Geometry: final body of the model. Coordinates: model frame, mm. Face numbers are marked on the shaded views. A direction names the side the tool comes from. Give positions to 0.01 mm unless a question says otherwise; leave off trailing zeros. Write each loop counter-clockwise with the first axis right and the second up, starting at its lowest first coordinate (ties: lowest second). Pieces come first, ordered by that corner, then holes.
Q1. Cut plane D-D on z = 7.75. Return the cut outline in (x, y).
Q2. Cut plane C-C on x = 3.75. Return the cut outline in (y, z), plus the area to 3 significant figures.
Q3. Pin query (flat end, axial travel): pin 1 (2 mm diameter, centred on x = 4.5, y = 0, fed in from +Z); pin 2 (2 mm diameter, centred on x = 6.5, y = 3.5, fed in from +Z). Return the tip coordinate at first contact, or that it passes through.
Q4. Draft query along Z for the marked faces 3, 4 and 5. Return one class per face: pulls with the +Z half, pulls with the -Z half, needs draft (parallel to the pull), parting line crosses it, or undercut.
Q5. Line query: L1, parallel to X at y = -0.75, z = 10; L2, parallel to Z at x = 5.75, y = 4; L3, parallel to Z at x = 1, y = 3.75. Output: solid intervals per line, ascending.
Q6. Reachability of the marked faces 1 and 2 from +Z, -Z, +X, -X, +Y, -Y: full face, straight path, thin tool, end or side. Return the list, or none.
Q7. Cut plane B-B on z = 13.75. Return the cut outline in (x, y), plus the area to 3 significant figures.
Q8. Cut plane A-A on y = 0.25. Return the cut outline in (x, z).
```python
from build123d import *

# Parameters (mm, degrees)
SKETCH1_R           = 6
BOSS_EXTRUDE1_DEPTH = 2
SKETCH2_R           = 4.5
BOSS_EXTRUDE2_DEPTH = 6
SKETCH3_R           = 3
CUT_EXTRUDE1_DEPTH  = 11
SKETCH4_W           = 17.898398612
SKETCH4_H           = 8.444372679
CUT_EXTRUDE2_DEPTH  = 11


with BuildPart() as part:
    # Sketch1 → Boss-Extrude1 (new body)
    with BuildSketch(Plane(origin=(0, 0, 0), x_dir=(0, 0, -1), z_dir=(1, 0, 0))):
        with Locations((-10.366970779, 4.315662044)):
            Circle(SKETCH1_R)
    extrude(amount=BOSS_EXTRUDE1_DEPTH)

    # Sketch2 → Boss-Extrude2 (add)
    with BuildSketch(Plane(origin=(2, 0, 0), x_dir=(0, 0, -1), z_dir=(1, 0, 0))):
        with Locations((-10.366970779, 4.315662044)):
            Circle(SKETCH2_R)
    extrude(amount=BOSS_EXTRUDE2_DEPTH)

    # Sketch3 → Cut-Extrude1 (cut)
    with BuildSketch(Plane(origin=(8, 0, 0), x_dir=(0, 0, -1), z_dir=(1, 0, 0))):
        with Locations((-10.366970779, 4.315662044)):
            Circle(SKETCH3_R)
    extrude(amount=-CUT_EXTRUDE1_DEPTH, mode=Mode.SUBTRACT)

    # Sketch4 → Cut-Extrude2 (cut)
    with BuildSketch(Plane(origin=(8, 0, 0), x_dir=(0, 0, -1), z_dir=(1, 0, 0))):
        with Locations((-9.724464162, 8.537848384)):
            Rectangle(SKETCH4_W, SKETCH4_H)
    extrude(amount=-CUT_EXTRUDE2_DEPTH, mode=Mode.SUBTRACT)


solid = part.part
```
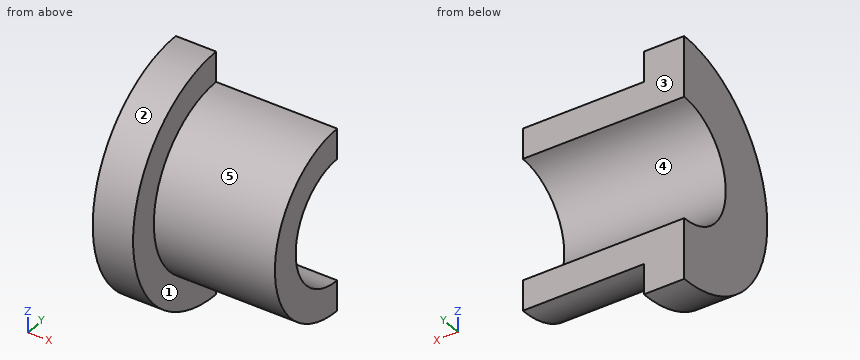
Data:
1. outline: (0, -1.08) - (2, -1.08) - (2, 0.65) - (8, 0.65) - (8, 2.85) - (0, 2.85) - close
2. outline: (4.32, 5.87) - (4.32, 7.37) arc R3 cw to (4.32, 13.37) - (4.32, 14.87) arc R4.5 ccw to start
2. area: 17.7 mm2
3. pin 1: stops at z = 13.41
3. pin 2: stops at z = 14.87
4. face 3: needs draft
4. face 4: undercut
4. face 5: parting line crosses it
5. L1: x = 0 to 2
5. L2: z = 5.88 to 7.38, 13.35 to 14.86
5. L3: z = 4.39 to 7.42, 13.31 to 16.34
6. face 1: +X, -Y
6. face 2: +X, -X, -Y
7. outline: (0, -0.64) - (2, -0.64) - (2, 1.35) - (8, 1.35) - (8, 4.32) - (0, 4.32) - close
7. area: 27.7 mm2
8. outline: (0, 5.95) - (2, 5.95) - (2, 8.44) - (8, 8.44) - (8, 12.3) - (2, 12.3) - (2, 14.78) - (0, 14.78) - close
